Verification items for the finished model (mm, model axes). A direction names the side the tool comes from. Give positions to 0.01 mm unless a question says otherwise; leave off trailing zeros. Loops run counter-clockwise (first coordinate to the right, second up) from the corner with the lowest first, then second, coordinate; pieces in that order, holes last. Notation, with made-up numbers: M 7.25,45.5 L 25.25,45.5 A28 ccw 25.25,72.5 Z; hole C 15.5,71.5 d5. An arc over 180 degrees is marked long. Answer in a Markdown table with one row per item.
```python
from build123d import *
from build123d.topology import SkipClean

# Parameters (mm, degrees)
EXTRUDE1_DEPTH               = 3.81
SKETCH8_R                    = 2.413
EXTRUDE8_DEPTH               = 3.81
SKETCH6_R                    = 5.715
EXTRUDE6_DEPTH               = 2.413
SKETCH4_R                    = 0.254
EXTRUDE4_DEPTH               = 6.731
SKETCH5_R                    = 1.0033
EXTRUDE5_DEPTH               = 2.794
FILLET2_R                    = 0.889
CHAMFER1_SIZE                = 0.635
SKETCH7_R                    = 0.381
EXTRUDE7_DEPTH               = 13.109035428
CHAMFER3_SIZE                = 0.635
EXTRUDE9_DEPTH               = 0.381
EXTRUDE10_DEPTH              = 1.397
EXTRUDE11_DEPTH              = 6.731
CIRPATTERN1_COUNT            = 8
EXTRUDE12_DEPTH              = 6.731
CHAMFER4_SIZE                = 0.381
CHAMFER4_SIZE2               = 0.659911358
EXTRUDE13_DEPTH              = 0.6604
CUT_REVOLVE1_ANGLE           = 130
CUT_REVOLVE1_OTHER_WAY_ANGLE = 90
BOSS_EXTRUDE1_DEPTH          = 6.071088642
CUT_EXTRUDE1_DEPTH           = 0.838688642
CHAMFER5_SIZE                = 0.1016
CHAMFER6_SIZE                = 0.3048


with BuildPart() as part:
    # Sketch1 → Extrude1 (new body)
    with BuildSketch(Plane.XY):
        with BuildLine():
            Line((-1.242889362, 3.556), (-1.813523477, 0.319773119))
            ThreePointArc((-1.813523477, 0.319773119), (0, -1.8415), (1.813523477, 0.319773119))
            Line((1.813523477, 0.319773119), (1.242889362, 3.556))
            Line((1.242889362, 3.556), (-1.242889362, 3.556))
        make_face()
    extrude(amount=EXTRUDE1_DEPTH)

    # Sketch8 → Extrude8 (add)
    with BuildSketch(Plane.XY.offset(3.81)):
        with Locations(Location((0, 0, 0), (0, 0, 129.743387424))):
            Circle(SKETCH8_R)
    extrude(amount=EXTRUDE8_DEPTH)

    # Sketch6 → Extrude6 (add)
    with BuildSketch(Plane.XY.offset(3.81)):
        Circle(SKETCH6_R)
    extrude(amount=EXTRUDE6_DEPTH)

    # Sketch4 → Extrude4 (cut)
    with BuildSketch(Plane.XY.offset(7.62)):
        Circle(SKETCH4_R)
    extrude(amount=-EXTRUDE4_DEPTH, mode=Mode.SUBTRACT)

    # Sketch5 → Extrude5 (add)
    with BuildSketch(Plane(origin=(0, 0, 0), x_dir=(-1, 0, 0), z_dir=(0, 0, -1))):
        with Locations(Location((0, 0, 0), (0, 0, 180))):
            Circle(SKETCH5_R)
    extrude(amount=EXTRUDE5_DEPTH)

    # Fillet2
    fillet2_edges = [part.edges().sort_by_distance(p)[0] for p in [
        (1.242889362, 3.556, 1.905),
        (-1.242889362, 3.556, 1.905),
    ]]
    fillet(fillet2_edges, radius=FILLET2_R)

    # Chamfer1
    chamfer1_edges = [part.edges().sort_by_distance(p)[0] for p in [
        (-5.715, 0, 3.81),
    ]]
    chamfer(chamfer1_edges, length=CHAMFER1_SIZE)

    # Sketch7 → Extrude7 (cut, through all)
    with BuildSketch(Plane.XY.offset(6.223)):
        with Locations((-1.150450655, -4.293540298)):
            Circle(SKETCH7_R)
    extrude(amount=-EXTRUDE7_DEPTH, mode=Mode.SUBTRACT)

    # Chamfer3
    chamfer3_edges = [part.edges().sort_by_distance(p)[0] for p in [
        (-5.715, 0, 6.223),
    ]]
    chamfer(chamfer3_edges, length=CHAMFER3_SIZE)

    # Sketch9 → Extrude9 (add)
    with BuildSketch(Plane(origin=(0, 0, 0), x_dir=(-1, 0, 0), z_dir=(0, 0, -1))):
        with BuildLine():
            Line((-0.3175, 3.302), (0.3175, 3.302))
            ThreePointArc((0.3175, 3.302), (0.586907684, 3.190407684), (0.6985, 2.921))
            Line((0.6985, 2.921), (0.6985, 0))
            Line((0.6985, 0), (-0.6985, 0))
            Line((-0.6985, 0), (-0.6985, 2.921))
            ThreePointArc((-0.6985, 2.921), (-0.586907684, 3.190407684), (-0.3175, 3.302))
        make_face()
    extrude(amount=EXTRUDE9_DEPTH)

    # Sketch11 → Extrude10 (cut)
    with BuildSketch(Plane(origin=(0, 0, 3.81), x_dir=(-1, 0, 0), z_dir=(0, 0, -1))):
        with BuildLine():
            Line((1.868871145, -3.575119808), (3.096912551, -4.803161214))
            Line((3.096912551, -4.803161214), (3.096912551, -5.713418243))
            Line((3.096912551, -5.713418243), (0.134450655, -5.713418243))
            Line((0.134450655, -5.713418243), (0.134450655, -4.293540298))
            ThreePointArc((0.134450655, -4.293540298), (0.761644288, -3.354878693), (1.868871145, -3.575119808))
        make_face()
    extrude(amount=-EXTRUDE10_DEPTH, mode=Mode.SUBTRACT)

    # Sketch17 → Extrude11 (cut)
    with BuildSketch(Plane.XY.offset(7.62)):
        with BuildLine():
            Line((0, 0), (0, 0.8128))
            ThreePointArc((0, 0.8128), (0.077181384, 0.80912723), (0.153665255, 0.798142111))
            ThreePointArc((0.153665255, 0.798142111), (0.281884616, 0.680529664), (0.455713955, 0.673029443))
            ThreePointArc((0.455713955, 0.673029443), (0.517563871, 0.626714831), (0.574736392, 0.574736392))
            Line((0.574736392, 0.574736392), (0, 0))
        make_face()
    extrude11 = extrude(amount=-EXTRUDE11_DEPTH, mode=Mode.SUBTRACT)

    # CirPattern1: Extrude11 ×8 about axis
    cirpattern1_axis = Axis((0, 0, 0), (0, 0, 1))
    for i in range(1, CIRPATTERN1_COUNT):
        add(extrude11.rotate(cirpattern1_axis, i * 360 / CIRPATTERN1_COUNT), mode=Mode.SUBTRACT)

    # Sketch18 → Extrude12 (add)
    with BuildSketch(Plane.XY.offset(7.62)):
        Polygon((-0.539167209, 0.608229037), (0.811331666, 0.048834087), (0.986294531, 0.471231809), (-0.364204343, 1.030626759), align=None)
    extrude(amount=-EXTRUDE12_DEPTH)

    # Chamfer4
    chamfer4_edges = [part.edges().sort_by_distance(p)[0] for p in [
        (0.136082229, 0.328531562, 7.62),
    ]]
    chamfer4_side = [part.faces().sort_by_distance(p)[0] for p in [
        (1.499116567, -1.802914954, 7.62),
    ]]
    chamfer(chamfer4_edges, length=CHAMFER4_SIZE, length2=CHAMFER4_SIZE2, reference=chamfer4_side[0])

    # Sketch19 → Extrude13 (cut)
    with SkipClean():  # the faces are left unmerged after this step: merging them gives an invalid solid
        with BuildSketch(Plane.XY.offset(7.62)):
            with BuildLine():
                Line((0.811331666, 0.048834087), (-0.539167209, 0.608229037))
                ThreePointArc((-0.539167209, 0.608229037), (-0.311045094, -0.750929284), (0.811331666, 0.048834087))
            make_face()
        extrude(amount=-EXTRUDE13_DEPTH, mode=Mode.SUBTRACT)

    # Sketch20 → Cut-Revolve1 (revolve, cut)
    with SkipClean():  # the faces are left unmerged after this step: merging them gives an invalid solid
        with BuildSketch(Plane(origin=(0, 0, 0), x_dir=(0, 0, -1), z_dir=(1, 0, 0))):
            Polygon((-6.9596, -0.8128), (-6.9596, 0), (-6.1468, 0), align=None)
        revolve(axis=Axis((0, 0, 7.389643883), (0, 0, -1)), revolution_arc=CUT_REVOLVE1_ANGLE, mode=Mode.SUBTRACT)

    # Sketch20 → Cut-Revolve1 other way (revolve, cut)
    with SkipClean():  # the faces are left unmerged after this step: merging them gives an invalid solid
        with BuildSketch(Plane(origin=(0, 0, 0), x_dir=(0, 0, -1), z_dir=(1, 0, 0))):
            Polygon((-6.9596, -0.8128), (-6.9596, 0), (-6.1468, 0), align=None)
        revolve(axis=Axis((0, 0, 7.389643883), (0, 0, 1)), revolution_arc=CUT_REVOLVE1_OTHER_WAY_ANGLE, mode=Mode.SUBTRACT)

    # Sketch21 → Boss-Extrude1 (add)
    with SkipClean():  # the faces are left unmerged after this step: merging them gives an invalid solid
        with BuildSketch(Plane.XY.offset(6.960088642)):
            with BuildLine():
                Line((-0.459893976, 0.575392988), (-0.539167209, 0.608229037))
                ThreePointArc((-0.539167209, 0.608229037), (-0.311045094, -0.750929284), (0.811331666, 0.048834087))
                Line((0.811331666, 0.048834087), (0.732058433, 0.081670135))
                ThreePointArc((0.732058433, 0.081670135), (-0.281884616, -0.680529664), (-0.459893976, 0.575392988))
            make_face()
        extrude(amount=-BOSS_EXTRUDE1_DEPTH)

    # Sketch22 → Cut-Extrude1 (cut)
    with SkipClean():  # the faces are left unmerged after this step: merging them gives an invalid solid
        with BuildSketch(Plane.XY.offset(6.960088642)):
            with BuildLine():
                Line((-0.459893976, 0.575392988), (-0.539167209, 0.608229037))
                ThreePointArc((-0.539167209, 0.608229037), (-0.311045094, -0.750929284), (0.811331666, 0.048834087))
                Line((0.811331666, 0.048834087), (0.732058433, 0.081670135))
                ThreePointArc((0.732058433, 0.081670135), (-0.281884616, -0.680529664), (-0.459893976, 0.575392988))
            make_face()
        extrude(amount=-CUT_EXTRUDE1_DEPTH, mode=Mode.SUBTRACT)

    # Chamfer5
    # the kernel refuses this chamfer: 0.1016 mm, written as the material it takes off along each edge
    with BuildSketch(Plane(origin=(0, 0, 6.1214), x_dir=(-0.3826834323650876, -0.9238795325112875, 0), z_dir=(0.9238795325112875, -0.3826834323650876, 0))) as chamfer5_piece_1_section:
        Polygon((0.7366 + CHAMFER5_SIZE, 0), (0.7366, CHAMFER5_SIZE), (0.7366, 0), align=None)
    chamfer5_piece_1 = revolve(axis=Axis((0, 0, 6.1214), (0, 0, -1)), revolution_arc=45, mode=Mode.PRIVATE)
    chamfer5_piece_1 = chamfer5_piece_1 & Plane(origin=(0, 0, 6.085965336), x_dir=(-0.6633454831704748, 0.74831328329606, 0), z_dir=(0, 0, 1)) * Cylinder(0.8128, 4, mode=Mode.PRIVATE)
    add(chamfer5_piece_1, mode=Mode.SUBTRACT)
    with BuildSketch(Plane(origin=(0, 0, 6.1214), x_dir=(0.3826834323650712, -0.9238795325112945, 0), z_dir=(0.9238795325112945, 0.3826834323650712, 0))) as chamfer5_piece_2_section:
        Polygon((0.7366 + CHAMFER5_SIZE, 0), (0.7366, CHAMFER5_SIZE), (0.7366, 0), align=None)
    chamfer5_piece_2 = revolve(axis=Axis((0, 0, 6.1214), (0, 0, -1)), revolution_arc=45, mode=Mode.PRIVATE)
    chamfer5_piece_2 = chamfer5_piece_2 & Plane(origin=(0, 0, 6.085965336), x_dir=(-0.6633454831704748, 0.74831328329606, 0), z_dir=(0, 0, 1)) * Cylinder(0.8128, 4, mode=Mode.PRIVATE)
    add(chamfer5_piece_2, mode=Mode.SUBTRACT)
    with BuildSketch(Plane(origin=(0, 0, 6.1214), x_dir=(-0.9238795325112938, -0.3826834323650728, 0), z_dir=(0.3826834323650728, -0.9238795325112938, 0))) as chamfer5_piece_3_section:
        Polygon((0.7366 + CHAMFER5_SIZE, 0), (0.7366, CHAMFER5_SIZE), (0.7366, 0), align=None)
    chamfer5_piece_3 = revolve(axis=Axis((0, 0, 6.1214), (0, 0, -1)), revolution_arc=45, mode=Mode.PRIVATE)
    chamfer5_piece_3 = chamfer5_piece_3 & Plane(origin=(0, 0, 6.085965336), x_dir=(-0.6633454831704748, 0.74831328329606, 0), z_dir=(0, 0, 1)) * Cylinder(0.8128, 4, mode=Mode.PRIVATE)
    add(chamfer5_piece_3, mode=Mode.SUBTRACT)
    with BuildSketch(Plane(origin=(0, 0, 6.1214), x_dir=(-0.9238795325112764, 0.3826834323651145, 0), z_dir=(-0.3826834323651145, -0.9238795325112764, 0))) as chamfer5_piece_4_section:
        Polygon((0.7366 + CHAMFER5_SIZE, 0), (0.7366, CHAMFER5_SIZE), (0.7366, 0), align=None)
    chamfer5_piece_4 = revolve(axis=Axis((0, 0, 6.1214), (0, 0, -1)), revolution_arc=49.190233443, mode=Mode.PRIVATE)
    chamfer5_piece_4 = chamfer5_piece_4 & Plane(origin=(0, 0, 6.085613455), x_dir=(-0.6633454831704748, 0.74831328329606, 0), z_dir=(0, 0, 1)) * Cylinder(0.8128, 4, mode=Mode.PRIVATE)
    chamfer5_piece_4 = split(chamfer5_piece_4, bisect_by=Plane(origin=(-0.544175649, 0.610303601, 6.085613455), z_dir=(-0.38268343236508656, -0.9238795325112882, 0)), keep=Keep.TOP, mode=Mode.PRIVATE)
    add(chamfer5_piece_4, mode=Mode.SUBTRACT)
    with BuildSketch(Plane(origin=(0, 0, 6.1214), x_dir=(0.9238795325112772, -0.3826834323651127, 0), z_dir=(0.3826834323651127, 0.9238795325112772, 0))) as chamfer5_piece_5_section:
        Polygon((0.7366 + CHAMFER5_SIZE, 0), (0.7366, CHAMFER5_SIZE), (0.7366, 0), align=None)
    chamfer5_piece_5 = revolve(axis=Axis((0, 0, 6.1214), (0, 0, -1)), revolution_arc=45, mode=Mode.PRIVATE)
    chamfer5_piece_5 = chamfer5_piece_5 & Plane(origin=(0, 0, 6.085965336), x_dir=(-0.6633454831704748, 0.74831328329606, 0), z_dir=(0, 0, 1)) * Cylinder(0.8128, 4, mode=Mode.PRIVATE)
    add(chamfer5_piece_5, mode=Mode.SUBTRACT)
    with BuildSketch(Plane(origin=(0, 0, 6.1214), x_dir=(0.8934479656215565, 0.44916670928142266, 0), z_dir=(-0.44916670928142266, 0.8934479656215565, 0))) as chamfer5_piece_6_section:
        Polygon((0.7366 + CHAMFER5_SIZE, 0), (0.7366, CHAMFER5_SIZE), (0.7366, 0), align=None)
    chamfer5_piece_6 = revolve(axis=Axis((0, 0, 6.1214), (0, 0, -1)), revolution_arc=49.190233443, mode=Mode.PRIVATE)
    chamfer5_piece_6 = chamfer5_piece_6 & Plane(origin=(0, 0, 6.085613455), x_dir=(-0.6633454831704748, 0.74831328329606, 0), z_dir=(0, 0, 1)) * Cylinder(0.8128, 4, mode=Mode.PRIVATE)
    chamfer5_piece_6 = split(chamfer5_piece_6, bisect_by=Plane(origin=(0.816340106, 0.046759523, 6.085613455), z_dir=(-0.38268343236508556, -0.9238795325112885, 0)), keep=Keep.TOP, mode=Mode.PRIVATE)
    add(chamfer5_piece_6, mode=Mode.SUBTRACT)

    # Chamfer6
    chamfer6_edges = [part.edges().sort_by_distance(p)[0] for p in [
        (-0.311045094, -0.750929284, 7.62),
    ]]
    chamfer(chamfer6_edges, length=CHAMFER6_SIZE)


solid = part.part
```
Item 1: Go/stop test with flat-tipped pins: pin 1 (0.5 mm diameter, centred on x = 0, z = 2, fed in from +Y); pin 2 (1.5 mm diameter, centred on y = 3.5, z = 4.5, fed in from -X); pin 3 (6 mm diameter, centred on x = -3.5, z = 4, fed in from +Y); pin 4 (3 mm diameter, centred on y = -4, z = -0.5, fed in from -X). Record where each tip stops, or that it passes through.
Reported:
| item | result |
|---|---|
| pin 1 | stops at y = 3.56 |
| pin 2 | stops at x = -5.01 |
| pin 3 | stops at y = 5.69 |
| pin 4 | passes through |
Item 2: Scan lines: L1, parallel to X at y = 0, z = 6.65; L2, parallel to Z at x = 3.5, y = -0.25; L3, parallel to Z at x = 0, y = -2. Record each from-to range of solid material in increasing order. Write a range as [from, to].
Reported:
| item | result |
|---|---|
| L1 | x = [-2.41, -0.81], [0.81, 2.41] |
| L2 | z = [3.81, 6.22] |
| L3 | z = [3.81, 7.62] |
Item 3: Tool access check on faces 4 (the cylindrical face through (-0.1, -1, -1.4)), 5 (the cylindrical face through (-1.075, 3.342, 1.932)), 6 (the flat face through (1.596, 1.553, 1.878)). Record the directions out of +Z, -Z, +X, -X, +Y, -Y that give a thin tool (end or side, any length) a straight path to the whole face; none if there is none.
Reported:
| item | result |
|---|---|
| face 4 | -Z |
| face 5 | -Z, -X, +Y |
| face 6 | -Z, +X, +Y |
Item 4: Sectioned sample at B-B (z = -2). Record the cut outline in (x, y).
Reported:
| item | result |
|---|---|
| outline | C 0,0 d2.01 |
Item 5: Release check for a two-part mould opening along Y. For faces 1 (the flat face through (0, 3.556, 2)), 2 (the conical face through (1.66, 4.92, 3.92)), 3 (the flat face through (0, 0, 0.889)) record: released by +Y, released by -Y, zero draft, split by the parting line, or undercut.
Reported:
| item | result |
|---|---|
| face 1 | released by +Y |
| face 2 | split by the parting line |
| face 3 | undercut |
Item 6: Sectioned sample at A-A (z = 3). Record the cut outline in (x, y), and give its area (3 significant figures).
Reported:
| item | result |
|---|---|
| outline | M -1.81,0.32 A1.84 ccw long 1.81,0.32 L 1.37,2.82 A0.89 ccw 0.5,3.56 L -0.5,3.56 A0.89 ccw -1.37,2.82 Z; hole M -0.46,0.58 A0.74 ccw long 0.73,0.08 Z |
| area | 14.8 mm^2 |
